```python
from build123d import *

# Parameters (mm, degrees)
SKETCH_0_R         = 210
SKETCH_0_R_2       = 7.5
PAD_DEPTH          = 10
PAD001_DEPTH       = 20
POLARPATTERN_COUNT = 6


with BuildPart() as part:
    with BuildSketch(Plane.YZ):
        Circle(SKETCH_0_R)
        Circle(SKETCH_0_R_2, mode=Mode.SUBTRACT)
    extrude(amount=-PAD_DEPTH)

    with BuildSketch(Plane.YZ):
        with BuildLine():
            Line((113.541139, 176.659021), (17.320508, 10))
            Line((209.76177, 10), (17.320508, 10))
            ThreePointArc((209.76177, 10), (181.865335, 105), (113.541139, 176.659021))
        make_face()
    pad001 = extrude(amount=PAD001_DEPTH)

    # PolarPattern: Pad001 ×6 about axis
    polarpattern_axis = Axis((0, 0, 0), (1, 0, 0))
    for i in range(1, POLARPATTERN_COUNT):
        add(pad001.rotate(polarpattern_axis, i * 360 / POLARPATTERN_COUNT))


solid = part.part
```
Source: CAD feature listing. Evaluate the final solid. Frame: model axes, mm. A direction names the side the tool comes from. Coordinates: 2 decimals unless noted, no trailing zeros. Loops run counter-clockwise (first coordinate to the right, second up) from the corner with the lowest first, then second, coordinate; pieces in that order, holes last. Notation, with made-up numbers: (25, 80.25) -> (63, 80.25) arc R31 ccw to (63, 112.25) -> close; hole circle Ø5 at (-20, 43). An arc over 180 degrees is marked (long way). One line per item, written item: value. Start each with the question number.
Q1. Contact query for flat-ended pins moving along their axis: P1, Ø8, axis at x = 0, y = -25, coming from the -Z side; P2, Ø10, axis at x = -6.5, z = 113, coming from the +Y side; P3, Ø19.5, axis at y = 0, z = 0, coming from the +X side. Output: stop coordinate, or through.
Q2. Section query B-B, the plane z = 0. Return the cut outline in (x, y).
Q3. Section query D-D, the plane z = -139.5. Return the cut outline in (x, y), and give its area (3 significant figures).
Q4. Set-up query: faces 3 (the face through (20, -122, 59)), 4 (the face through (10, -115, 10)), 5 (the face through (9.86, 66.104, -94.496)). Return all of +Z, -Z, +X, -X, +Y, -Y with unobstructed straight access to the full face (end or side cutting, diameter ignored); none if empty.
Q5. Mould query, pull axis Y, two halves, no side actions, for faces 1 (the face through (9.86, 48.784, 104.496)), 2 (the face through (10, 115, -10)). Classes: pulls with the +Y half, pulls with the -Y half, needs draft (parallel to the pull), parting line crosses it, or undercut.
Q6. Line query: line 1 along Z through (x, y) = (-3, 0); line 2 along Z through (x, y) = (15.25, 79.5); line 3 along Y through (x, z) = (12.5, -147.5). Output: solid intervals per line, ascending.
Q7. Section query A-A, the plane x = 13.75. Return the cut outline in (y, z), and give its area (3 significant figures).
Q8. Section query C-C, the plane y = 12.5. Return the cut outline in (x, z), and give its area (3 significant figures).
Results:
1. P1: z = -208.95
1. P2: y = 180.1
1. P3: x = 0
2. outline: (-10, -210) -> (0, -210) -> (0, -7.5) -> (-10, -7.5) -> close; (-10, 7.5) -> (0, 7.5) -> (0, 210) -> (-10, 210) -> close
3. outline: (-10, -156.97) -> (20, -156.97) -> (20, -92.09) -> (0, -92.09) -> (0, -68.99) -> (20, -68.99) -> (20, 68.99) -> (0, 68.99) -> (0, 92.09) -> (20, 92.09) -> (20, 156.97) -> (-10, 156.97) -> close
3. area: 8,490 mm^2
4. face 3: +Z, -Z, +X, +Y, -Y
4. face 4: +X, +Y, -Y
4. face 5: +X
5. face 1: undercut
5. face 2: needs draft
6. line 1: -210 to -7.5, 7.5 to 210
6. line 2: -194.37 to -157.7, -117.7 to -10, 10 to 117.7, 157.7 to 194.37
6. line 3: -149.48 to -96.71, -73.61 to 73.61, 96.71 to 149.48
7. outline: (-209.76, -10) arc R210 ccw to (-113.54, -176.66) -> (-17.32, -10) -> close; (-209.76, 10) -> (-17.32, 10) -> (-113.54, 176.66) arc R210 ccw to start; (-96.22, -186.66) arc R210 ccw to (96.22, -186.66) -> (0, -20) -> close; (-96.22, 186.66) -> (0, 20) -> (96.22, 186.66) arc R210 ccw to start; (17.32, -10) -> (113.54, -176.66) arc R210 ccw to (209.76, -10) -> close; (17.32, 10) -> (209.76, 10) arc R210 ccw to (113.54, 176.66) -> close
7. area: 114,000 mm^2
8. outline: (-10, -209.63) -> (20, -209.63) -> (20, -41.65) -> (0, -41.65) -> (0, 41.65) -> (20, 41.65) -> (20, 209.63) -> (-10, 209.63) -> close
8. area: 10,900 mm^2
